Could you check a few things on this model? Use its own coordinates, in mm. Give positions to 0.01 mm unless a question says otherwise; leave off trailing zeros. Write each loop counter-clockwise with the first axis right and the second up, starting at its lowest first coordinate (ties: lowest second). Pieces come first, ordered by that corner, then holes. Notation, with made-up numbers: M 57,41 L 110,41 A24 ccw 110,68 Z; hole C 63.5,64.5 d6. An arc over 180 degrees is marked long. Answer as a JSON object with one key per item and string values. Group by question number.
```python
from build123d import *

# Parameters (mm, degrees)
SKETCH_1_R          = 6
EXTRUDE_1_DEPTH     = 5
FILLET_1_R          = 5
FILLET_2_R          = 75
FILLET_3_R          = 5
EXTRUDE_2_DEPTH     = 5
CUT_EXTRUDE_2_DEPTH = 160.415234704


with BuildPart() as part:
    # Эскиз1 → Бобышка-Вытянуть1 (new body)
    with BuildSketch(Plane(origin=(0, 0, 0), x_dir=(0, 0, -1), z_dir=(1, 0, 0))):
        with BuildLine():
            Line((126.237664014, 58.886284382), (98.821729218, -16.438377404))
            Line((98.821729218, -16.438377404), (-151.178270782, -25.884067346))
            Line((-151.178270782, -25.884067346), (-77.345590471, -3.080194644))
            Line((-77.345590471, -3.080194644), (-77.345590471, -13.087329783))
            Line((-77.345590471, -13.087329783), (75.539410437, -7.310912522))
            Line((75.539410437, -7.310912522), (90.975731778, 35.100031802))
            ThreePointArc((90.975731778, 35.100031802), (108.905022115, 46.550907327), (126.237664014, 58.886284382))
        make_face()
        with Locations((103.870185422, 30.698515365)):
            Circle(SKETCH_1_R, mode=Mode.SUBTRACT)
    extrude(amount=EXTRUDE_1_DEPTH)

    # Скругление1
    fillet_1_edges = [part.edges().sort_by_distance(p)[0] for p in [
        (2.5, -13.087329783, 77.345590471),
    ]]
    fillet(fillet_1_edges, radius=FILLET_1_R)

    # Скругление2
    # the kernel refuses this fillet: 75 mm, written as the material it adds along each edge
    with BuildSketch(Plane(origin=(0, -7.310912522, -75.539410437), x_dir=(0, -0.037755820465347284, 0.9992869948223027), z_dir=(1, 0, 0))) as fillet_2_piece_1:
        with BuildLine():
            CenterArc((50.223853574, -75), FILLET_2_R, 90, 63.724056715)
            Line((-17.026575163, -41.797894123), (0, 0))
            Line((0, 0), (50.223853574, 0))
        make_face()
    extrude(amount=5)
    # the kernel refuses this fillet: 75 mm, written as the material it takes off along each edge
    with BuildSketch(Plane(origin=(-126.080854452, -16.438377404, -98.821729218), x_dir=(0, -0.03775582046534733, 0.9992869948223025), z_dir=(1, 0, 0))) as fillet_2_2_piece_1:
        with BuildLine():
            CenterArc((FILLET_2_R * 0.672431223743, -FILLET_2_R), FILLET_2_R, 90, 67.836236553)
            Line((-FILLET_2_R * 0.253678140212, -FILLET_2_R * 0.622744852924), (0, 0))
            Line((0, 0), (FILLET_2_R * 0.672431223743, 0))
        make_face()
    extrude(amount=257.161708904, mode=Mode.SUBTRACT)

    # Скругление3
    fillet_3_edges = [part.edges().sort_by_distance(p)[0] for p in [
        (2.5, 58.886284382, -126.237664014),
    ]]
    fillet(fillet_3_edges, radius=FILLET_3_R)

    # Эскиз4 → Бобышка-Вытянуть2 (add)
    with BuildSketch(Plane(origin=(5, 0, 0), x_dir=(0, 0, -1), z_dir=(1, 0, 0))):
        with BuildLine():
            Line((-105.187577254, -24.146412021), (-31.354896943, -1.342539319))
            Line((-31.354896943, -1.342539319), (-31.354896943, -6.15719309))
            ThreePointArc((-31.354896943, -6.15719309), (-29.890430849, -9.692726996), (-26.354896943, -11.15719309))
            Line((-26.354896943, -11.15719309), (-31.354896943, -21.356809597))
            Line((-31.354896943, -21.356809597), (-105.187577254, -24.146412021))
        make_face()
    extrude(amount=-EXTRUDE_2_DEPTH)

    # Эскиз5 → Вырез-Вытянуть2 (cut, through all)
    with BuildSketch(Plane(origin=(5, 0, 0), x_dir=(0, 0, -1), z_dir=(1, 0, 0))):
        Polygon((-38.471521652, -3.540571454), (-146.983243384, -37.055371114), (-175.325798577, -14.870573448), (-65.732340229, 27.748343591), align=None)
    extrude(amount=-CUT_EXTRUDE_2_DEPTH, mode=Mode.SUBTRACT)


solid = part.part
```
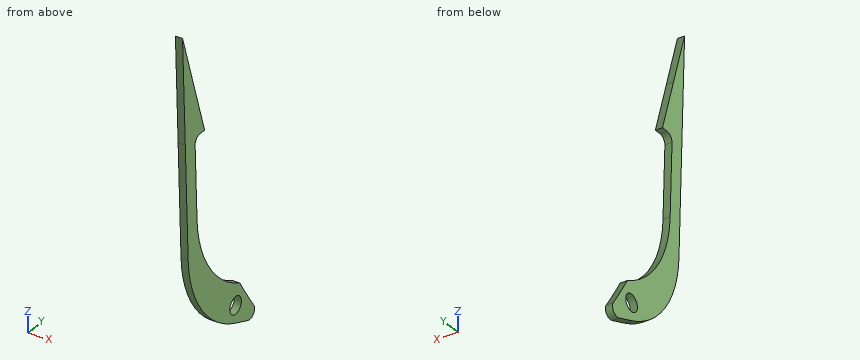
1) If we section it at C-C, the plane y = 27.5: List the corners of the cut face in (x, z) for me, plus the area to 3 significant figures.
2) If we section it at A-A, the plane z = -103: List the corners of the cut face in (x, y) for me, plus the area to 3 significant figures.
3) I'm going to push flat-ended pins straight in: pin 1 (2 mm diameter, centred on x = 1, z = 3, fed in from -Y); pin 2 (1.5 mm diameter, centred on x = 2.5, y = 33, fed in from +Z); pin 3 (1.4 mm diameter, centred on x = 2.5, y = -4.5, fed in from -Z); pin 4 (6 mm diameter, centred on y = 31, z = -86, fed in from -X). Where does each tip first touch, or does it pass through?
4) Please list where these lines run through material, in increasing order: line 1 along Z through (x, y) = (0.25, 33.5); line 2 along Y through (x, z) = (4.1, 47); line 3 along Y through (x, z) = (1.2, -49). Write a range as from..to.
5) If we section it at D-D, the plane y = 7.5: List the corners of the cut face in (x, z) for me.
Taken from the geometry:
{
 "1": {"outline": "M 0,-114.72 L 5,-114.72 L 5,-108.95 L 0,-108.95 Z; M 0,-98.79 L 5,-98.79 L 5,-87.04 L 0,-87.04 Z", "area": "87.6 mm²"},
 "2": {"outline": "M 0,8.34 L 5,8.34 L 5,24.76 L 0,24.76 Z; M 0,36.64 L 5,36.64 L 5,42.64 L 0,42.64 Z", "area": "112 mm²"},
 "3": {"pin 1": "y = -20.32", "pin 2": "z = -89.63", "pin 3": "z = -90.05", "pin 4": "x = 0"},
 "4": {"line 1": "-117..-109.18, -98.56..-90.24", "line 2": "-21.95..-6.17", "line 3": "-18.32..-4.43"},
 "5": {"outline": "M 0,-102.28 L 5,-102.28 L 5,-69.78 L 0,-69.78 Z"}
}
